Part model, mm, in its own coordinate system. A direction names the side the tool comes from. Round coordinates to 2 decimals unless told otherwise and drop trailing zeros. Loops run counter-clockwise (first coordinate to the right, second up) from the corner with the lowest first, then second, coordinate; pieces in that order, holes last. Notation, with made-up numbers: M 14.5,-14 L 72.5,-14 A26 ccw 72.5,9 Z; hole C 12.5,40.25 d10. An arc over 180 degrees is marked long. Put each result on its own line as item: value. Start each with the question number.
1) Probe line 1 along Y through (x, z) = (-6, 2); line 2 along Z through (x, y) = (4.25, 0.75); line 3 along Z through (x, y) = (10.75, 3.5). List the from-to ranges inside material, lowest first.
2) Slice it at B-B on x = 0. Give the cut face in (y, z), then the cut area to 3 significant figures.
3) Pull direction Y, two halves, no side cores. Call faces 4 (the cylindrical face through (-5.87, -7.24, 1.69)), 5 (the cylindrical face through (2.539, -1.947, -20.305)), 6 (the flat face through (0, 0, -23.91)): +Y half, -Y half, draft (parallel to the pull), parting line (faces both ways), or undercut.
4) Slice it at C-C on z = -7. Give the cut face in (x, y).
5) Drop flat-ended pins along their axis: pin 1 Ø3.5 at (x, y) = (9.525, 0) entering from +Z; pin 2 Ø10 at (y, z) = (-6.5, 3.5) entering from -X; pin 3 Ø10 at (y, z) = (5, -11.5) entering from -X; pin 4 Ø12.5 at (x, y) = (2, -6) entering from -Z. Give the stop position or say it passes through.
6) Which spindle directions (+Z, -Z, +X, -X, +Y, -Y) get a long thin tool onto all of the face, cutting with end or side? Do faces 1 (the cylindrical face through (-5.87, 9.26, 1.69)), 2 (the cylindrical face through (-2.539, -1.947, 6.835)), 3 (the cylindrical face through (6, 0, -8)). Say none if no direction does.
7) Slice it at D-D on z = 2. Give the cut face in (x, y) (1 decimal), then the cut area to 3 significant figures.
8) Slice it at A-A on y = 0. Give the cut face in (x, z) (3 decimals).
```python
from build123d import *

# Parameters (mm, degrees)
SKETCH1_R           = 12.7
BOSS_EXTRUDE1_DEPTH = 3.33
SKETCH2_R           = 3.2
BOSS_EXTRUDE2_DEPTH = 7.11
SKETCH3_R           = 6
BOSS_EXTRUDE3_DEPTH = 16.8
SKETCH4_R           = 3.2
BOSS_EXTRUDE4_DEPTH = 7.11
SKETCH5_R           = 1.5
CUT_EXTRUDE1_DEPTH  = 7.11


with BuildPart() as part:
    # Sketch1 → Boss-Extrude1 (new body)
    with BuildSketch(Plane.XY):
        Circle(SKETCH1_R)
    extrude(amount=BOSS_EXTRUDE1_DEPTH)

    # Sketch2 → Boss-Extrude2 (add)
    with BuildSketch(Plane.XY.offset(3.33)):
        Circle(SKETCH2_R)
    extrude(amount=BOSS_EXTRUDE2_DEPTH)

    # Sketch3 → Boss-Extrude3 (add)
    with BuildSketch(Plane(origin=(0, 0, 0), x_dir=(-1, 0, 0), z_dir=(0, 0, -1))):
        Circle(SKETCH3_R)
    extrude(amount=BOSS_EXTRUDE3_DEPTH)

    # Sketch4 → Boss-Extrude4 (add)
    with BuildSketch(Plane(origin=(0, 0, -16.8), x_dir=(-1, 0, 0), z_dir=(0, 0, -1))):
        Circle(SKETCH4_R)
    extrude(amount=BOSS_EXTRUDE4_DEPTH)

    # Sketch5 → Cut-Extrude1 (cut)
    with BuildSketch(Plane.XY.offset(3.33)):
        with Locations((9.525, 0)):
            Circle(SKETCH5_R)
        with Locations((-4.7625, -8.248891971)):
            Circle(SKETCH5_R)
        with Locations((-4.7625, 8.248891971)):
            Circle(SKETCH5_R)
    extrude(amount=-CUT_EXTRUDE1_DEPTH, mode=Mode.SUBTRACT)


solid = part.part
```
Recorded:
1. line 1: y = -11.19 to -9.1, -7.4 to 7.4, 9.1 to 11.19
1. line 2: z = -16.8 to 3.33
1. line 3: z = 0 to 3.33
2. outline: M -12.7,0 L -6,0 L -6,-16.8 L -3.2,-16.8 L -3.2,-23.91 L 3.2,-23.91 L 3.2,-16.8 L 6,-16.8 L 6,0 L 12.7,0 L 12.7,3.33 L 3.2,3.33 L 3.2,10.44 L -3.2,10.44 L -3.2,3.33 L -12.7,3.33 Z
2. area: 377 mm2
3. face 4: undercut
3. face 5: parting line
3. face 6: draft
4. outline: C 0,0 d12
5. pin 1: stops at z = 3.33
5. pin 2: stops at x = -12.61
5. pin 3: stops at x = -6
5. pin 4: stops at z = -23.91
6. face 1: +Z, -Z
6. face 2: +Z
6. face 3: -Z
7. outline: C 0,0 d25.4; hole C -4.8,-8.2 d3; hole C -4.8,8.2 d3; hole C 9.5,0 d3
7. area: 486 mm2
8. outline: M -12.7,0 L -6,0 L -6,-16.8 L -3.2,-16.8 L -3.2,-23.91 L 3.2,-23.91 L 3.2,-16.8 L 6,-16.8 L 6,0 L 8.025,0 L 8.025,3.33 L 3.2,3.33 L 3.2,10.44 L -3.2,10.44 L -3.2,3.33 L -12.7,3.33 Z; M 11.025,0 L 12.7,0 L 12.7,3.33 L 11.025,3.33 Z
